from build123d import *

# Parameters (mm, degrees)
F1_DEPTH = 25


with BuildPart() as f1:
    # F0 (on Front) → F1 (new body)
    with BuildSketch(Plane.XZ):
        Polygon((151.666667, -140), (200, 150), (195, 150), (195, 140), (185, 140), (185, 150), (175, 150), (175, 140), (165, 140), (165, 150), (155, 150), (155, 140), (145, 140), (145, 150), (135, 150), (135, 140), (125, 140), (125, 150), (115, 150), (115, 140), (105, 140), (105, 150), (95, 150), (95, 140), (85, 140), (85, 150), (75, 150), (75, 140), (65, 140), (65, 150), (55, 150), (55, 140), (45, 140), (45, 150), (35, 150), (35, 140), (25, 140), (25, 150), (15, 150), (15, 140), (5, 140), (5, 150), (0, 150), (-5, 150), (-5, 140), (-15, 140), (-15, 150), (-25.5, 150), (-25.5, 140), (-35.5, 140), (-35.5, 150), (-46, 150), (-46, 140), (-56, 140), (-56, 150), (-66.5, 150), (-66.5, 140), (-76.5, 140), (-76.5, 150), (-87, 150), (-87, 140), (-97, 140), (-97, 150), (-107.5, 150), (-107.5, 140), (-117.5, 140), (-117.5, 150), (-128, 150), (-128, 140), (-138, 140), (-138, 150), (-148.5, 150), (-148.5, 140), (-158.5, 140), (-158.5, 150), (-169, 150), (-169, 140), (-179, 140), (-179, 150), (-189.5, 150), (-189.5, 140), (-198.333333, 140), (-151.666667, -140), (-148.5, -140), (-148.5, -150), (-138, -150), (-138, -140), (-128, -140), (-128, -150), (-117.5, -150), (-117.5, -140), (-107.5, -140), (-107.5, -150), (-97, -150), (-97, -140), (-87, -140), (-87, -150), (-76.5, -150), (-76.5, -140), (-66.5, -140), (-66.5, -150), (-56, -150), (-56, -140), (-46, -140), (-46, -150), (-35.5, -150), (-35.5, -140), (-25.5, -140), (-25.5, -150), (-15, -150), (-15, -140), (-5, -140), (-5, -150), (0, -150), (5, -150), (5, -140), (15, -140), (15, -150), (25, -150), (25, -140), (35, -140), (35, -150), (45, -150), (45, -140), (55, -140), (55, -150), (65, -150), (65, -140), (75, -140), (75, -150), (85, -150), (85, -140), (95, -140), (95, -150), (105, -150), (105, -140), (115, -140), (115, -150), (125, -150), (125, -140), (135, -140), (135, -150), (145, -150), (145, -140), align=None)
    extrude(amount=F1_DEPTH)


solid = f1.part
The listing builds one solid part. Answer for the finished solid, in the listing's coordinates (mm). A direction names the side the tool comes from. Give positions to 0.01 mm unless a question says otherwise; leave off trailing zeros. Loops run counter-clockwise (first coordinate to the right, second up) from the corner with the lowest first, then second, coordinate; pieces in that order, holes last.
Item 1: Determine the mould class of faces 4 (the flat face through (-2, 0, 2)), 5 (the flat face through (-117.5, -12, -145)) for opening direction X: +X half, -X half, draft (parallel to the pull), parting line (faces both ways), or undercut.
Derived:
face 4: draft
face 5: undercut
Item 2: A cutting plane is placed at A-A (x = 70). Give the vertices of the cut face in (y, z).
Derived:
outline: (-25, -140) - (0, -140) - (0, 140) - (-25, 140) - close
Item 3: A cutting plane is placed at B-B (z = 48). Give the vertices of the cut face in (x, y), then the cut area to 3 significant figures.
Derived:
outline: (-183, -25) - (183, -25) - (183, 0) - (-183, 0) - close
area: 9,150 mm2
Item 4: Each of these flat-tipped pins is pushed along its axis until it touches: pin 1 Ø12 at (y, z) = (-20, -108) entering from +X; pin 2 Ø5 at (x, y) = (88, -7.5) entering from -Z; pin 3 Ø10 at (y, z) = (-7, 20.5) entering from +X. Where does it stop, or does it pass through?
Derived:
pin 1: stops at x = 158
pin 2: stops at z = -140
pin 3: stops at x = 179.25
Item 5: A tool of negligible diameter and unlimited length cuts with its end or side. For faces 1 (the flat face through (170, -12, 140)), 2 (the flat face through (-133, -12, -140)), 3 (the flat face through (140, -12, -150)), from which of +Z, -Z, +X, -X, +Y, -Y can it reach the whole face along a straight path? Write none if from no direction.
Derived:
face 1: +Z, +Y, -Y
face 2: -Z, +Y, -Y
face 3: -Z, +X, -X, +Y, -Y
Item 6: Find the intervals of material crossed by line 1 along Z through (x, y) = (7, -2.5); line 2 along X through (y, z) = (-16.75, -33.5); line 3 along X through (y, z) = (-4, -116.5), in increasing order.
Derived:
line 1: z = -140 to 140
line 2: x = -169.42 to 169.42
line 3: x = -155.58 to 155.58
